Here's the drawing with two shaded views (mm, measured from the low corner). I have some questions. Round coordinates to 2 decimals unless told otherwise and drop trailing zeros. Order: outer loops, then holes, each group sorted by start corner. A loop starts at its lowest first (then second) coordinate and runs counter-clockwise, first axis right, second up.
Q1. If we section it at A-A (y = 0.55): Please give me the cut outline in (x, z).
Q2. If we section it at C-C (x = 35.5): Please give me the cut outline in (y, z).
Q3. If I drill on line 1 (Z direction, x = 78.5, y = 0.85); line 2 (Z direction, x = 69, y = 0.25), over which ranges is the centre line in solid material (lowest first)?
Q4. If we section it at B-B (z = 15): Please give me the cut outline in (x, y).
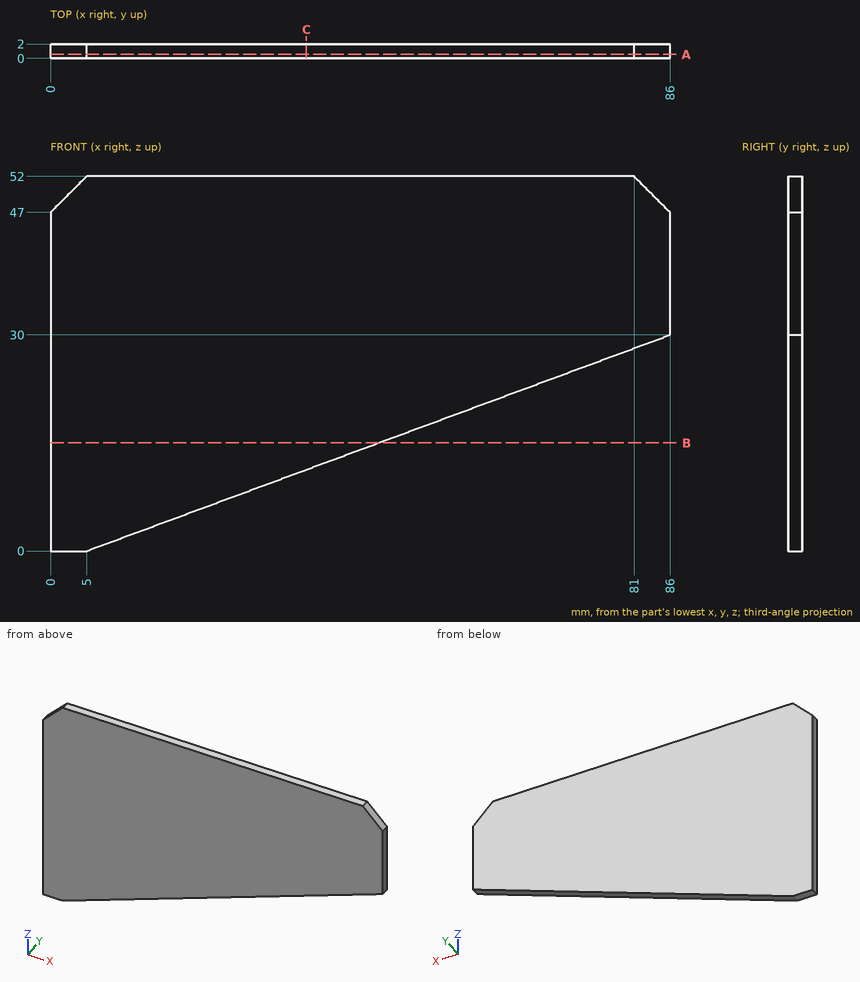
Solution:
1. outline: (0, 0) - (5, 0) - (86, 30) - (86, 47) - (81, 52) - (5, 52) - (0, 47) - close
2. outline: (0, 11.3) - (2, 11.3) - (2, 52) - (0, 52) - close
3. line 1: z = 27.22 to 52
3. line 2: z = 23.7 to 52
4. outline: (0, 0) - (45.5, 0) - (45.5, 2) - (0, 2) - close
